Design review of the part built by this model. Coordinates are the model's own, in mm. Give positions to 0.01 mm unless a question says otherwise; leave off trailing zeros. Write each loop counter-clockwise with the first axis right and the second up, starting at its lowest first coordinate (ties: lowest second). Pieces come first, ordered by that corner, then holes.
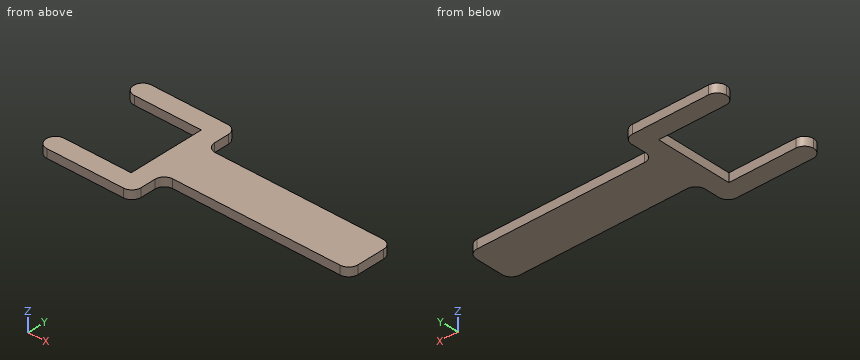
```python
from build123d import *

# Parameters (mm, degrees)
F1_DEPTH = 4.7625
F2_R     = 5.07999


# Not quite as in the source:
# - a fillet or chamfer is up to 0.001 mm smaller than in the source, because OpenCascade refuses the exact size
# - a length typed as a fraction of an inch, garbled in the dataset ("3 / 203.2 mm" for 3/8 in), is restored


with BuildPart() as f1:
    # F0 (on Top) → F1 (new body)
    with BuildSketch(Plane.XY):
        Polygon((41.656, 0), (0, 0), (0, -10.16), (51.816, -10.16), (51.816, 8.128), (153.416, 8.128), (153.416, 33.528), (51.816, 33.528), (51.816, 51.816), (0, 51.816), (0, 41.656), (41.656, 41.656), align=None)
    extrude(amount=F1_DEPTH)

    # F2 (radius 5.08 in the source; OpenCascade refuses exactly that, so slightly less here)
    f2_edges = [f1.edges().sort_by_distance(p)[0] for p in [
        (0, 41.656, 2.38125),
        (0, 51.816, 2.38125),
        (0, 0, 2.38125),
        (0, -10.16, 2.38125),
        (51.816, -10.16, 2.38125),
        (51.816, 8.128, 2.38125),
        (51.816, 33.528, 2.38125),
        (51.816, 51.816, 2.38125),
        (153.416, 33.528, 2.38125),
        (153.416, 8.128, 2.38125),
    ]]
    fillet(f2_edges, radius=F2_R)


solid = f1.part
```
(1) To check wall thickness, follow L1, parallel to Y at x = 20, z = 4.4; L2, parallel to Y at x = 64.5, z = 3.5; L3, parallel to X at y = 3, z = 0.5. State the ranges of each line that lie inside material, in increasing order.
Resolved:
L1: y = -10.16 to 0, 41.66 to 51.82
L2: y = 8.13 to 33.53
L3: x = 41.66 to 51.82
(2) Consider section C-C, the plane x = 82. Give the boundary of the cut face in (y, z), then the cut area to 3 significant figures.
Resolved:
outline: (8.13, 0) - (33.53, 0) - (33.53, 4.76) - (8.13, 4.76) - close
area: 121 mm2
(3) Consider section D-D, the plane y = 26.5. Give the boundary of the cut face in (x, z).
Resolved:
outline: (41.66, 0) - (153.42, 0) - (153.42, 4.76) - (41.66, 4.76) - close
(4) Consider section A-A, the plane x = 16.5. Give the boundary of the cut face in (y, z), then the cut area to 3 significant figures.
Resolved:
outline: (-10.16, 0) - (0, 0) - (0, 4.76) - (-10.16, 4.76) - close; (41.66, 0) - (51.82, 0) - (51.82, 4.76) - (41.66, 4.76) - close
area: 96.8 mm2
(5) Clearance check with flat-ended pins moving along their axes: P1, Ø1, axis at x = 54, y = -2.5, coming from the -Z side; P2, Ø2.5, axis at y = 0, z = 3.5, coming from the +X side. State where each tip first meets the part, or that it passes through.
Resolved:
P1: passes through
P2: stops at x = 51.82
